Here's the drawing with two shaded views (mm, measured from the low corner). I have some questions. A direction names the side the tool comes from. Give positions to 0.01 mm unless a question says otherwise; leave off trailing zeros. Write each loop counter-clockwise with the first axis right and the second up, starting at its lowest first coordinate (ties: lowest second). Pieces come first, ordered by that corner, then holes. Notation, with made-up numbers: M 66.25,-33 L 106.25,-33 A6 cw 106.25,-25 Z; hole C 6.25,55.5 d2. An arc over 180 degrees is marked long. Use one line per item in the form item = value.
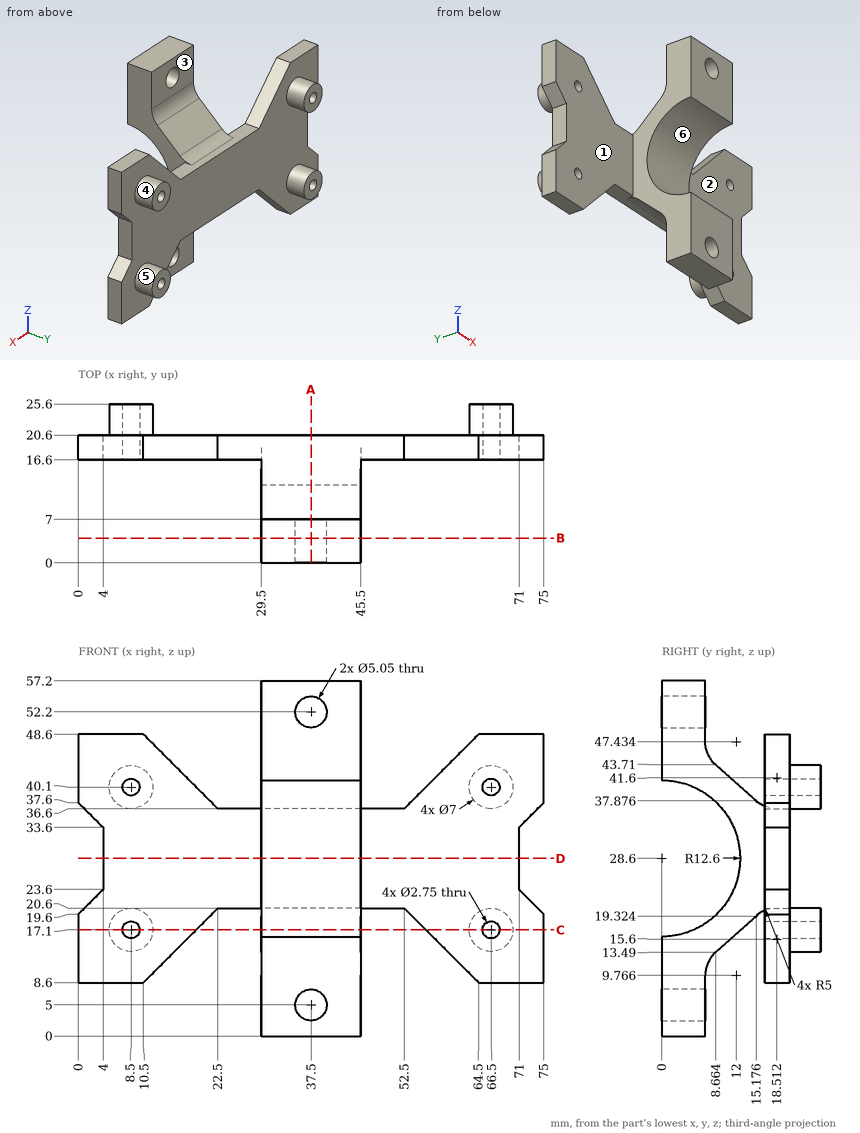
1) For the marked faces 1, 2, 3 and 4, which set-ups out of +Z, -Z, +X, -X, +Y, -Y let a thin tool reach every point of the face, with its end or its side?
Checked values:
face_1 = +Z, -Z, -X, -Y
face_2 = +Z, -Z, +X, -Y
face_3 = +Z, +X, -X, +Y
face_4 = +Y
2) If I drill on L1, parallel to X at y = 23.75, z = 40.1 (1 decimal); L2, parallel to Z at x = 8.5, y = 19.5 (1 decimal); L3, parallel to Z at x = 8.5, y = 21.75 (1 decimal), over which ranges is the centre line in solid material (lowest first)?
Checked values:
L1 = 5 to 7.1, 9.9 to 12, 63 to 65.1, 67.9 to 70
L2 = 8.6 to 15.7, 18.5 to 38.7, 41.5 to 48.6
L3 = 13.6 to 15.7, 18.5 to 20.6, 36.6 to 38.7, 41.5 to 43.6
3) I want a section at A-A, the plane x = 37.5. Please give me the cut outline in (y, z) (1 decimal).
Checked values:
outline = M 0,0 L 7,0 L 7,2.5 L 0,2.5 Z; M 0,7.5 L 7,7.5 L 7,9.8 A5 cw 8.7,13.5 L 15.2,19.3 A5 cw 18.5,20.6 L 20.6,20.6 L 20.6,36.6 L 18.5,36.6 A5 cw 15.2,37.9 L 8.7,43.7 A5 cw 7,47.4 L 7,49.7 L 0,49.7 L 0,41.2 A12.6 cw 0,16 Z; M 0,54.7 L 7,54.7 L 7,57.2 L 0,57.2 Z
4) Thinking about a two-plate mould opening in X: for the marked faces 5 and 6, which applies, released by +X, released by -X, zero draft, split by the parting line, or undercut?
Checked values:
face_5 = undercut
face_6 = zero draft
5) I want a section at C-C, the plane z = 17.1. Please give me the cut outline in (x, y) (1 decimal).
Checked values:
outline = M 0,16.6 L 7.1,16.6 L 7.1,25.6 L 5,25.6 L 5,20.6 L 0,20.6 Z; M 9.9,16.6 L 19,16.6 L 19,20.6 L 12,20.6 L 12,25.6 L 9.9,25.6 Z; M 29.5,5.1 L 45.5,5.1 L 45.5,12.7 L 29.5,12.7 Z; M 56,16.6 L 65.1,16.6 L 65.1,25.6 L 63,25.6 L 63,20.6 L 56,20.6 Z; M 67.9,16.6 L 75,16.6 L 75,20.6 L 70,20.6 L 70,25.6 L 67.9,25.6 Z
6) I want a section at D-D, the plane z = 28.6. Please give me the cut outline in (x, y).
Checked values:
outline = M 4,16.6 L 29.5,16.6 L 29.5,12.6 L 45.5,12.6 L 45.5,16.6 L 71,16.6 L 71,20.6 L 4,20.6 Z
7) I want a section at B-B, the plane y = 4. Count the separate pieces of the cut face and the enclosed holes in it, plus the area to 3 significant figures.
Checked values:
separate_pieces = 2
enclosed_holes = 2
area = 493 mm2
8) For pin 1 Ø4.5 at (x, y) = (68, 19) entering from -Z; pin 2 Ø4.5 at (x, z) = (66.5, 17.1) entering from -Y; pin 3 Ø9.5 at (y, z) = (11.5, 19.5) entering from -X, each with a flat end and sliding along its axis, tell me the tip position at first contact or that it passes through.
Checked values:
pin_1 = 8.6
pin_2 = 16.6
pin_3 = 29.5
